```python
from build123d import *

# Parameters (mm, degrees)
CROQUIS1_R              = 42.5
SALIENTE_EXTRUIR1_DEPTH = 25
CROQUIS2_R              = 1.5
CROQUIS2_R_2            = 2
CROQUIS2_RX             = 3.5
CROQUIS2_RY             = 3
CORTAR_EXTRUIR1_DEPTH   = 25


with BuildPart() as part:
    # Croquis1 → Saliente-Extruir1 (new body)
    with BuildSketch(Plane(origin=(0, 0, 0), x_dir=(1, 0, 0), z_dir=(0, 1, 0))):
        with Locations(Location((0, 0, 0), (0, 0, 270))):
            Circle(CROQUIS1_R)
    extrude(amount=SALIENTE_EXTRUIR1_DEPTH)

    # Croquis2 → Cortar-Extruir1 (cut)
    with BuildSketch(Plane(origin=(0, 25, 0), x_dir=(1, 0, 0), z_dir=(0, 1, 0))):
        with Locations(Location((0, 30.405, 0), (0, 0, 270))):
            Circle(CROQUIS2_R)
        with Locations(Location((30.405, 0, 0), (0, 0, 270))):
            Circle(CROQUIS2_R)
        with Locations(Location((0, -30.405, 0), (0, 0, 270))):
            Circle(CROQUIS2_R)
        with Locations(Location((-30.405, 0, 0), (0, 0, 270))):
            Circle(CROQUIS2_R)
        with Locations(Location((-38, 0, 0), (0, 0, 270))):
            Circle(CROQUIS2_R_2)
        with Locations(Location((38, 0, 0), (0, 0, 270))):
            Circle(CROQUIS2_R_2)
        with Locations(Location((25.455844123, 25.455844123), (0, 0, -48.360743663))):
            Ellipse(CROQUIS2_RX, CROQUIS2_RY)
    extrude(amount=-CORTAR_EXTRUIR1_DEPTH, mode=Mode.SUBTRACT)


solid = part.part
```
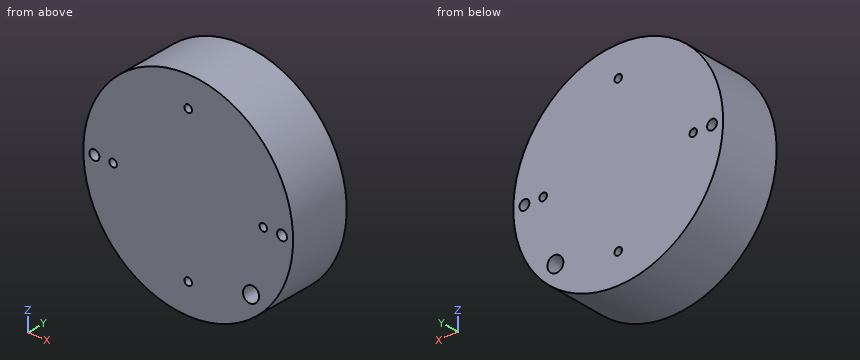
Verification items for the finished model (mm, model axes). Coordinates: 2 decimals unless noted, no trailing zeros. Order: outer loops, then holes, each group sorted by start corner. A loop starts at its lowest first (then second) coordinate and runs counter-clockwise, first axis right, second up. Notation, with made-up numbers: (17.5, 18.5) -> (67.5, 18.5) arc R36 cw to (67.5, 57.5) -> close; hole circle Ø1 at (58, 47.25). An arc over 180 degrees is marked (long way). Answer as CSV lines item,"result". Start each with the question number.
1) Gauge pin test, flat ends, axial feed: pin 1 Ø2 at (y, z) = (15.5, -29.5) entering from -X; pin 2 Ø6 at (y, z) = (13.5, -22.5) entering from -X; pin 3 Ø8 at (y, z) = (10, 12) entering from -X; pin 4 Ø1.8 at (x, z) = (30.405, 0) entering from -Y. Record the tip position at first contact, or that the pin passes through.
2) Cross-section at A-A, the plane x = 0. Record the boundary of the cut face in (y, z) (3 decimals), then the cut area to 4 significant figures.
3) Cross-section at D-D, the plane z = 37.5. Record the boundary of the cut face in (x, y).
4) Material ranges on L1, parallel to X at y = 8.25, z = 0 (3 decimals); L2, parallel to Z at x = 26, y = 12.5; L3, parallel to X at y = 8.25, z = -31.5, recorded low to high. Write a range as [from, to].
5) Cross-section at B-B, the plane z = 0. Record the boundary of the cut face in (x, y) (3 decimals), then the cut area to 4 significant figures.
6) Cross-section at C-C, the plane x = -38. Record the boundary of the cut face in (y, z).
Conclusion:
1,pin 1,"stops at x = -31.53"
1,pin 2,"stops at x = -37.76"
1,pin 3,"stops at x = -41.74"
1,pin 4,"passes through"
2,outline,"(0, -42.5) -> (25, -42.5) -> (25, -31.905) -> (0, -31.905) -> close; (0, -28.905) -> (25, -28.905) -> (25, 28.905) -> (0, 28.905) -> close; (0, 31.905) -> (25, 31.905) -> (25, 42.5) -> (0, 42.5) -> close"
2,area,"1,975 mm²"
3,outline,"(-20, 0) -> (20, 0) -> (20, 25) -> (-20, 25) -> close"
4,L1,"x = [-42.5, -40], [-36, -31.905], [-28.905, 28.905], [31.905, 36], [40, 42.5]"
4,L2,"z = [-33.62, -28.58], [-22.17, 33.62]"
4,L3,"x = [-28.53, -1.03], [1.03, 28.53]"
5,outline,"(-42.5, 0) -> (-40, 0) -> (-40, 25) -> (-42.5, 25) -> close; (-36, 0) -> (-31.905, 0) -> (-31.905, 25) -> (-36, 25) -> close; (-28.905, 0) -> (28.905, 0) -> (28.905, 25) -> (-28.905, 25) -> close; (31.905, 0) -> (36, 0) -> (36, 25) -> (31.905, 25) -> close; (40, 0) -> (42.5, 0) -> (42.5, 25) -> (40, 25) -> close"
5,area,"1,775 mm²"
6,outline,"(0, -19.03) -> (25, -19.03) -> (25, -2) -> (0, -2) -> close; (0, 2) -> (25, 2) -> (25, 19.03) -> (0, 19.03) -> close"
